Autodesk Inventor part; units mm, degrees
ref_plane "YZ Plane" through (0, 0, 0) normal (1, 0, 0) x (0, 1, 0)
ref_plane "XZ Plane" through (0, 0, 0) normal (0, 1, 0) x (-1, 0, 0)
ref_plane "XY Plane" through (0, 0, 0) normal (0, 0, 1) x (1, 0, 0)
sketch "Sketch1" plane through (0, 0, 0) normal (0, 0, 1) x (1, 0, 0)
  circle A0 centre (0, 0) radius 7.5
  circle A1 centre (0, 0) radius 2.985
  dimension "d0" = 15
  dimension "d1" = 5.97
extrude "Extrusion1" add sketch "Sketch1" along normal blind 14 contours A0 | A1
extrude "Extrusion2" cut sketch "Sketch1" along normal blind 10 contours A1
chamfer "Chamfer1" distance 1 distance2 13 1 edges at (-7.5, 0, 14) measured on face at (1.2064, -0.2974, 14)
fillet "Fillet1" radius 1 2 edges at (-6.5, 0, 14) (-7.5, 0, 0)
properties part number "Encoder Knobe"
The listing builds one solid part. Answer for the finished solid, in the listing's coordinates (mm). A direction names the side the tool comes from. Round coordinates to 2 decimals unless told otherwise and drop trailing zeros. Write each loop counter-clockwise with the first axis right and the second up, starting at its lowest first coordinate (ties: lowest second). Pieces come first, ordered by that corner, then holes. Notation, with made-up numbers: M -0.5,87 L 8.5,87 A13 cw 8.5,92 Z; hole C 28,75.5 d3. An arc over 180 degrees is marked long. Write each question's results on one line, items separated by ' | '. Start each with the question number.
Item 1: Flat-ended cylindrical pins translate along their axes: pin 1 Ø5 at (x, z) = (-2.5, 2) entering from +Y; pin 2 Ø1.5 at (x, z) = (4.5, 8) entering from +Y. Find the tip coordinate at first contact, or state that the pin passes through.
Item 2: A cutting plane is placed at B-B on z = 12.25. Write down the section's boundary in (x, y).
Item 3: A cutting plane is placed at A-A on z = 2.5. Write down the section's boundary in (x, y) (3 decimals).
Item 4: For a pull along Y with two mould halves and no side action, classify faces 3 (the face through (3, -2, 0)), 4 (the face through (6.5, 2.7, 7)), 5 (the face through (-0.647, 2.914, 4.93)) as pulls with the +Y half, pulls with the -Y half, needs draft (parallel to the pull), parting line crosses it, or undercut.
Item 5: For faces 1 (the face through (0, 0, 10)), 2 (the face through (0, 0, 14)), determine the directions among +Z, -Z, +X, -X, +Y, -Y from which every point of the face is accessible in a straight line to the end or side of a thin tool.
Item 6: A cutting plane is placed at C-C on z = 6. Write down the section's boundary in (x, y) (3 decimals).
Item 7: Straight lines are drawn through the part: L1, parallel to Z at x = 1, y = 2; L2, parallel to Y at x = -0.5, z = 7.5; L3, parallel to Y at x = 0, z = 5.75 (3 decimals). For each, find the intervals that lie inside material, in ascending order. Write a range as [from, to].
Check sheet entries:
1) pin 1: y = 7.49 | pin 2: y = 5.87
2) outline: C 0,0 d13.27
3) outline: C 0,0 d14.769; hole C 0,0 d5.97
4) face 3: needs draft | face 4: parting line crosses it | face 5: undercut
5) face 1: -Z | face 2: +Z, +X, -X, +Y, -Y
6) outline: C 0,0 d14.231; hole C 0,0 d5.97
7) L1: [10, 14] | L2: [-6.98, -2.94], [2.94, 6.98] | L3: [-7.135, -2.985], [2.985, 7.135]
